```python
from build123d import *

# Parameters (mm, degrees)
SKETCH4_W                = 42
SKETCH4_H                = 52
BOSS_EXTRUDE4_DEPTH      = 1.5
BOSS_EXTRUDE5_DEPTH      = 1.5
BOSS_EXTRUDE5_DEPTH_BACK = 0.0001
SKETCH5_W                = 205
SKETCH5_H                = 56.5
SKETCH8_W                = 1.5
SKETCH8_H                = 430
BOSS_EXTRUDE14_DEPTH     = 4
SKETCH7_W                = 205
SKETCH7_H                = 56.5
BOSS_EXTRUDE18_DEPTH     = 1.5
SKETCH9_W                = 433
SKETCH9_H                = 56.5
BOSS_EXTRUDE19_DEPTH     = 1.5
SKETCH15_R               = 2.1
CUT_EXTRUDE1_DEPTH       = 10
CUT_EXTRUDE2_START       = -10
SKETCH14_R               = 2.1
CUT_EXTRUDE2_DEPTH       = 10
CUT_EXTRUDE3_START       = -10
SKETCH12_R               = 2.1
CUT_EXTRUDE3_DEPTH       = 10
CUT_EXTRUDE4_START       = -10
SKETCH10_R               = 2.1
CUT_EXTRUDE4_DEPTH       = 10
CUT_EXTRUDE5_START       = -10
SKETCH11_R               = 2.1
CUT_EXTRUDE5_DEPTH       = 10
SKETCH17_W               = 42
SKETCH17_H               = 22
CUT_EXTRUDE6_DEPTH       = 10
SKETCH18_W               = 50.068809171
SKETCH18_H               = 30
CUT_EXTRUDE7_DEPTH       = 10
SKETCH19_R               = 1.75
CUT_EXTRUDE8_DEPTH       = 10
SKETCH23_W               = 7
SKETCH23_H               = 18
CUT_EXTRUDE10_DEPTH      = 31


with BuildPart() as part:
    # Sketch4 → Boss-Extrude4 (new body)
    with BuildSketch(Plane(origin=(0, 0, 0), x_dir=(1, 0, 0), z_dir=(0, 1, 0))):
        Polygon((139.373653762, 430), (344.373653762, 430), (344.373653762, 0), (139.373653762, 0), (139.373653762, 65), (139.373653762, 230), align=None)
        with Locations((200.373653762, 66)):
            Rectangle(SKETCH4_W, SKETCH4_H, mode=Mode.SUBTRACT)
    extrude(amount=BOSS_EXTRUDE4_DEPTH)

    # Sketch5 → Boss-Extrude5 (add, two sides: drawn at the far end of the back side and taken through both)
    with BuildSketch(Plane.XY.offset(-BOSS_EXTRUDE5_DEPTH_BACK)):
        with Locations((241.873653762, -26.75)):
            Rectangle(SKETCH5_W, SKETCH5_H)
    extrude(amount=BOSS_EXTRUDE5_DEPTH + BOSS_EXTRUDE5_DEPTH_BACK)

    # Sketch8 → Boss-Extrude14 (add)
    with BuildSketch(Plane(origin=(0, 1.5, 0), x_dir=(1, 0, 0), z_dir=(0, 1, 0))):
        with Locations((343.623653762, 215)):
            Rectangle(SKETCH8_W, SKETCH8_H)
    extrude(amount=BOSS_EXTRUDE14_DEPTH)

    # Sketch7 → Boss-Extrude18 (add)
    with BuildSketch(Plane(origin=(0, 0, -430), x_dir=(-1, 0, 0), z_dir=(0, 0, -1))):
        with Locations((-241.873653762, -26.75)):
            Rectangle(SKETCH7_W, SKETCH7_H)
    extrude(amount=BOSS_EXTRUDE18_DEPTH)

    # Sketch9 → Boss-Extrude19 (add)
    with BuildSketch(Plane.ZY.offset(-139.373653762)):
        with Locations((-215, -26.75)):
            Rectangle(SKETCH9_W, SKETCH9_H)
    extrude(amount=BOSS_EXTRUDE19_DEPTH)

    # Sketch15 → Cut-Extrude1 (cut)
    with BuildSketch(Plane(origin=(0, 0, -431.5), x_dir=(-1, 0, 0), z_dir=(0, 0, -1))):
        with Locations((-169.373653762, -25)):
            Circle(SKETCH15_R)
        with Locations((-149.373653762, -25)):
            Circle(SKETCH15_R)
        with Locations((-169.373653762, -45)):
            Circle(SKETCH15_R)
        with Locations((-149.373653762, -45)):
            Circle(SKETCH15_R)
    extrude(amount=-CUT_EXTRUDE1_DEPTH, mode=Mode.SUBTRACT)

    # Sketch14 → Cut-Extrude2 (cut)
    with BuildSketch(Plane.XY.offset(1.5).offset(CUT_EXTRUDE2_START)):
        with Locations(Location((169.373653762, -25, 0), (0, 0, 180))):
            Circle(SKETCH14_R)
    extrude(amount=CUT_EXTRUDE2_DEPTH, mode=Mode.SUBTRACT)

    # Sketch12 → Cut-Extrude3 (cut)
    with BuildSketch(Plane.XY.offset(1.5).offset(CUT_EXTRUDE3_START)):
        with Locations(Location((149.373653762, -25, 0), (0, 0, 180))):
            Circle(SKETCH12_R)
    extrude(amount=CUT_EXTRUDE3_DEPTH, mode=Mode.SUBTRACT)

    # Sketch10 → Cut-Extrude4 (cut)
    with BuildSketch(Plane.XY.offset(1.5).offset(CUT_EXTRUDE4_START)):
        with Locations(Location((169.373653762, -45, 0), (0, 0, 180))):
            Circle(SKETCH10_R)
    extrude(amount=CUT_EXTRUDE4_DEPTH, mode=Mode.SUBTRACT)

    # Sketch11 → Cut-Extrude5 (cut)
    with BuildSketch(Plane.XY.offset(1.5).offset(CUT_EXTRUDE5_START)):
        with Locations(Location((149.373653762, -45, 0), (0, 0, 180))):
            Circle(SKETCH11_R)
    extrude(amount=CUT_EXTRUDE5_DEPTH, mode=Mode.SUBTRACT)

    # Sketch17 → Cut-Extrude6 (cut)
    with BuildSketch(Plane(origin=(0, 1.5, 0), x_dir=(1, 0, 0), z_dir=(0, 1, 0))):
        with Locations((159.837104003, 175.311739833)):
            Rectangle(SKETCH17_W, SKETCH17_H)
    extrude(amount=-CUT_EXTRUDE6_DEPTH, mode=Mode.SUBTRACT)

    # Sketch18 → Cut-Extrude7 (cut)
    with BuildSketch(Plane.XY.offset(1.5)):
        with Locations((271.339249177, -26)):
            Rectangle(SKETCH18_W, SKETCH18_H)
    extrude(amount=-CUT_EXTRUDE7_DEPTH, mode=Mode.SUBTRACT)

    # Sketch19 → Cut-Extrude8 (cut)
    with BuildSketch(Plane.XY.offset(1.5)):
        with Locations((270.543410902, -5.5)):
            Circle(SKETCH19_R)
        with Locations((270.543410902, -45.5)):
            Circle(SKETCH19_R)
    extrude(amount=-CUT_EXTRUDE8_DEPTH, mode=Mode.SUBTRACT)

    # Sketch23 → Cut-Extrude10 (cut)
    with BuildSketch(Plane(origin=(0, 0, -431.5), x_dir=(-1, 0, 0), z_dir=(0, 0, -1))):
        with Locations((-340.873653762, -3.5)):
            Rectangle(SKETCH23_W, SKETCH23_H)
    extrude(amount=-CUT_EXTRUDE10_DEPTH, mode=Mode.SUBTRACT)


solid = part.part
```
Could you check a few things on this model? Use its own coordinates, in mm. A direction names the side the tool comes from. Round coordinates to 2 decimals unless told otherwise and drop trailing zeros. Loops run counter-clockwise (first coordinate to the right, second up) from the corner with the lowest first, then second, coordinate; pieces in that order, holes last. Notation, with made-up numbers: (57.5, 26.25) -> (81.5, 26.25) arc R33 ccw to (81.5, 61.25) -> close; hole circle Ø10 at (5.5, 83.25). An arc over 180 degrees is marked (long way). Put each result on its own line as item: value.
Q1. I want a section at A-A on x = 279. Write out the boundary of the cut face in (y, z), and give its area (3 significant figures).
Checks:
outline: (-55, -431.5) -> (1.5, -431.5) -> (1.5, 1.5) -> (-11, 1.5) -> (-11, 0) -> (0, 0) -> (0, -430) -> (-55, -430) -> close; (-55, 0) -> (-41, 0) -> (-41, 1.5) -> (-55, 1.5) -> close
area: 770 mm2
Q2. Thinking about a two-plate mould opening in Z: for faces 1 (the flat face through (243, -27, 1.5)), 2 (the flat face through (243, 0, -218)), 3 (the flat face through (243, 1.5, -218)), which applies, pulls with the +Z half, pulls with the -Z half, needs draft (parallel to the pull), parting line crosses it, or undercut?
Checks:
face 1: pulls with the +Z half
face 2: undercut
face 3: needs draft
Q3. Which directions (+Z, -Z, +X, -X, +Y, -Y) give clear straight access to the entire face, cutting with the end or side of a thin tool? Please do faces 4 (the flat face through (243, -27, -430)), 5 (the flat face through (137.874, -26, -218)), 6 (the flat face through (337.374, 0.2, -419.5)).
Checks:
face 4: +X, -Y
face 5: +Z, -Z, -X, +Y, -Y
face 6: -Z, +X, +Y
Q4. I want a section at B-B on z = -46.5. Write out the boundary of the cut face in (x, y), and give its area (3 significant figures).
Checks:
outline: (137.87, -55) -> (139.37, -55) -> (139.37, 0) -> (179.37, 0) -> (179.37, 1.5) -> (137.87, 1.5) -> close; (221.37, 0) -> (344.37, 0) -> (344.37, 5.5) -> (342.87, 5.5) -> (342.87, 1.5) -> (221.37, 1.5) -> close
area: 335 mm2
Q5. For pin 1 Ø11 at (y, z) = (-1.5, -177) entering from +X; pin 2 Ø6 at (x, z) = (241, -321.5) entering from +Y; pin 3 Ø11 at (y, z) = (-8, -417) entering from +X; pin 4 Ø1 at (x, z) = (251, -293.5) entering from -Y, each with a flat end and sliding along its axis, tell me the tip position at first contact or that it passes through.
Checks:
pin 1: x = 344.37
pin 2: y = 1.5
pin 3: x = 139.37
pin 4: y = 0
Q6. I want a section at C-C on x = 328.5. Write out the boundary of the cut face in (y, z), and give its area (3 significant figures).
Checks:
outline: (-55, -431.5) -> (1.5, -431.5) -> (1.5, 1.5) -> (-55, 1.5) -> (-55, 0) -> (0, 0) -> (0, -430) -> (-55, -430) -> close
area: 815 mm2
Q7. Please list where these lines run through material, in increasing order: line 1 (X direction, y = -45, z = 0.95); line 2 (Z direction, x = 216.5, y = -34); line 3 (X direction, y = -5, z = 1). Write a range as from..to.
Checks:
line 1: 137.87..147.27, 151.47..167.27, 171.47..268.87, 272.22..344.37
line 2: -431.5..-430, 0..1.5
line 3: 137.87..268.87, 272.22..344.37
Q8. I want a section at D-D on z = -375.5. Write out the boundary of the cut face in (x, y).
Checks:
outline: (137.87, -55) -> (139.37, -55) -> (139.37, 0) -> (344.37, 0) -> (344.37, 5.5) -> (342.87, 5.5) -> (342.87, 1.5) -> (137.87, 1.5) -> close
